Check sheet for the modelled part. Datum: model origin and axes. Units: mm. A direction names the side the tool comes from. Give positions to 0.01 mm unless a question says otherwise; leave off trailing zeros. Write each loop counter-clockwise with the first axis right and the second up, starting at its lowest first coordinate (ties: lowest second). Pieces come first, ordered by that corner, then holes. Notation, with made-up numbers: (19.25, 26) -> (53.25, 26) arc R13 cw to (53.25, 46) -> close; hole circle Ø2 at (-9.5, 56). An arc over 180 degrees is marked (long way). Answer as a JSON object with one key per item and string values.
from build123d import *

# Parameters (mm, degrees)
EXTRUDE_1_DEPTH     = 27
CUT_EXTRUDE_1_DEPTH = 1
CUT_EXTRUDE_4_DEPTH = 7
EXTRUDE_2_DEPTH     = 6.5


with BuildPart() as part:
    # 草圖1 → 填料-伸長1 (new body)
    with BuildSketch(Plane.XY):
        with BuildLine():
            Line((-32.2, 25), (-32.2, -36))
            Line((-32.2, -36), (-31.25, -36))
            Line((-31.25, -36), (-31.759558328, -37.4))
            Line((-31.759558328, -37.4), (-29.040441672, -37.4))
            Line((-29.040441672, -37.4), (-29.55, -36))
            Line((-29.55, -36), (-28.6, -36))
            Line((-28.6, -36), (-28.6, 25))
            ThreePointArc((-28.6, 25), (-25.378174593, 32.778174593), (-17.6, 36))
            Line((-17.6, 36), (17.6, 36))
            ThreePointArc((17.6, 36), (25.378174593, 32.778174593), (28.6, 25))
            Line((28.6, 25), (28.6, -36))
            Line((28.6, -36), (29.55, -36))
            Line((29.55, -36), (29.040441672, -37.4))
            Line((29.040441672, -37.4), (31.759558328, -37.4))
            Line((31.759558328, -37.4), (31.25, -36))
            Line((31.25, -36), (32.2, -36))
            Line((32.2, -36), (32.2, 25))
            ThreePointArc((32.2, 25), (27.923759005, 35.323759005), (17.6, 39.6))
            Line((17.6, 39.6), (-17.6, 39.6))
            ThreePointArc((-17.6, 39.6), (-27.923759005, 35.323759005), (-32.2, 25))
        make_face()
    extrude(amount=EXTRUDE_1_DEPTH)

    # 草圖4 → 除料-伸長1 (cut)
    with BuildSketch(Plane.XY.offset(3)):
        with BuildLine():
            Line((-28.6, -36), (-28.6, 25))
            ThreePointArc((-28.6, 25), (-25.378174593, 32.778174593), (-17.6, 36))
            Line((-17.6, 36), (17.6, 36))
            ThreePointArc((17.6, 36), (25.378174593, 32.778174593), (28.6, 25))
            Line((28.6, 25), (28.6, -36))
            Line((28.6, -36), (28.6, -37.4))
            Line((28.6, -37.4), (29.56, -37.4))
            Line((29.56, -37.4), (29.56, -36))
            Line((29.56, -36), (29.56, 25))
            ThreePointArc((29.56, 25), (26.056997103, 33.456997103), (17.6, 36.96))
            Line((17.6, 36.96), (-17.6, 36.96))
            ThreePointArc((-17.6, 36.96), (-26.056997103, 33.456997103), (-29.56, 25))
            Line((-29.56, 25), (-29.56, -36))
            Line((-29.56, -36), (-29.56, -37.4))
            Line((-29.56, -37.4), (-28.6, -37.4))
            Line((-28.6, -37.4), (-28.6, -36))
        make_face()
    extrude(amount=-CUT_EXTRUDE_1_DEPTH, mode=Mode.SUBTRACT)

    # 掃出2: sweep along a path in 草圖5
    with BuildLine(Plane.XY.offset(27)) as sweep_2_path:
        Line((-30.4, -36), (-30.4, 25))
        ThreePointArc((-30.4, 25), (-26.650966799, 34.050966799), (-17.6, 37.8))
        Line((-17.6, 37.8), (17.6, 37.8))
        ThreePointArc((17.6, 37.8), (26.650966799, 34.050966799), (30.4, 25))
        Line((30.4, 25), (30.4, -36))
    # 草圖7 → 掃出2 (sweep)
    with BuildSketch(Plane.XZ.offset(36)):
        with BuildLine():
            Line((-28.6, 27), (-32.2, 27))
            ThreePointArc((-32.2, 27), (-30.266904756, 31.666904756), (-25.6, 33.6))
            Line((-25.6, 33.6), (-25.6, 30))
            ThreePointArc((-25.6, 30), (-27.721320344, 29.121320344), (-28.6, 27))
        make_face()
    sweep(path=sweep_2_path.line)

    # 草圖9 → 除料-伸長4 (cut)
    with BuildSketch(Plane(origin=(0, 0, 0), x_dir=(-1, 0, 0), z_dir=(0, 0, -1))):
        Polygon((-5.85, 39.6), (-6.359558328, 38.2), (-3.640441672, 38.2), (-4.15, 39.6), align=None)
        Polygon((5.85, 39.6), (4.15, 39.6), (3.640441672, 38.2), (6.359558328, 38.2), align=None)
    extrude(amount=-CUT_EXTRUDE_4_DEPTH, mode=Mode.SUBTRACT)

    # 草圖10 → 填料-伸長2 (add, symmetric)
    with BuildSketch(Plane(origin=(0, 0, 0), x_dir=(0, 0, -1), z_dir=(1, 0, 0))):
        with BuildLine():
            Line((-5.9, 38.2), (-5.1, 38.2))
            ThreePointArc((-5.1, 38.2), (-5.5, 38.334643123), (-5.9, 38.2))
        make_face()
    extrude(amount=EXTRUDE_2_DEPTH, both=True)


solid = part.part
1. Sectioned sample at B-B, the plane z = 9. Enter the section's corners in (x, y).
Determined:
{"outline": "(-32.2, -36) -> (-31.25, -36) -> (-31.76, -37.4) -> (-29.04, -37.4) -> (-29.55, -36) -> (-28.6, -36) -> (-28.6, 25) arc R11 cw to (-17.6, 36) -> (17.6, 36) arc R11 cw to (28.6, 25) -> (28.6, -36) -> (29.55, -36) -> (29.04, -37.4) -> (31.76, -37.4) -> (31.25, -36) -> (32.2, -36) -> (32.2, 25) arc R14.6 ccw to (17.6, 39.6) -> (-17.6, 39.6) arc R14.6 ccw to (-32.2, 25) -> close"}
2. Sectioned sample at C-C, the plane x = -8. Enter the section's corners in (y, z).
Determined:
{"outline": "(33, 30) arc R3 cw to (36, 27) -> (36, 3) -> (36.96, 3) -> (36.96, 2) -> (36, 2) -> (36, 0) -> (39.6, 0) -> (39.6, 27) arc R6.6 ccw to (33, 33.6) -> close"}
3. Scan lines: L1, parallel to X at y = -30, z = 3.5; L2, parallel to X at y = -21.5, z = 28.5; L3, parallel to Y at x = 8.5, z = 15.5. Record each from-to range of solid material in increasing order. Write a range as [from, to].
Determined:
{"L1": "[-32.2, -28.6], [28.6, 32.2]", "L2": "[-32.03, -28.2], [28.2, 32.03]", "L3": "[36, 39.6]"}
4. Sectioned sample at A-A, the plane y = -18.5. Enter the section's corners in (x, z).
Determined:
{"outline": "(-32.2, 0) -> (-28.6, 0) -> (-28.6, 2) -> (-29.56, 2) -> (-29.56, 3) -> (-28.6, 3) -> (-28.6, 27) arc R3 cw to (-25.6, 30) -> (-25.6, 33.6) arc R6.6 ccw to (-32.2, 27) -> close; (25.6, 30) arc R3 cw to (28.6, 27) -> (28.6, 3) -> (29.56, 3) -> (29.56, 2) -> (28.6, 2) -> (28.6, 0) -> (32.2, 0) -> (32.2, 27) arc R6.6 ccw to (25.6, 33.6) -> close"}
5. Go/stop test with flat-tipped pins: P1, Ø1.8, axis at y = 0.5, z = 32, coming from the -X side; P2, Ø1.5, axis at x = 30.5, y = -36.5, coming from the +Z side; P3, Ø2, axis at x = -23.5, z = 10.5, coming from the +Y side; P4, Ø0.5, axis at x = 29, z = 1.5, coming from the -Y side. Record where each tip stops, or that it passes through.
Determined:
{"P1": "x = -30.77", "P2": "z = 31.97", "P3": "y = 38.75", "P4": "y = -37.4"}
6. Access from +Z, -Z, +X, -X, +Y, -Y to the whole of each face (thin tool, end or side, straight path). Record for faces 1 (the face through (26.149, 33.363, 2.507)), 2 (the face through (28.6, -5, 15)), 3 (the face through (0, 33, 32)).
Determined:
{"face 1": "-Y", "face 2": "-Z, -Y", "face 3": "+Z, -Z, -Y"}
